Here's how the part is built. I have some questions about the finished solid (model axes, mm). Face numbers are marked on the shaded views. A direction names the side the tool comes from. Give positions to 0.01 mm unless a question says otherwise; leave off trailing zeros. Loops run counter-clockwise (first coordinate to the right, second up) from the corner with the lowest first, then second, coordinate; pieces in that order, holes last. Notation, with made-up numbers: M 78,57 L 123,57 A33 cw 123,89 Z; hole C 35,39.5 d6. An arc over 180 degrees is marked long. Answer as CSV lines item,"result". Start each with the question number.
Item 1: I want a section at A-A on z = 22. List the corners of the cut face in (x, y) for me.
Item 2: If I drill on line 1 along Y through (x, z) = (-90, -13); line 2 along Y through (x, z) = (-90, -21); line 3 along Z through (x, y) = (-107, 9), over which ranges is the centre line in solid material (lowest first)? Write a range as from..to.
Item 3: Will these pins go through, and if not, where does the flat tip stop? P1, Ø1, axis at x = 39.5, z = -3, coming from the +Y side; P2, Ø2, axis at x = 87.5, z = -5, coming from the +Y side; P3, Ø5.5, axis at x = -3.5, z = -17, coming from the +Y side; P4, Ø20, axis at x = 90, y = 50, coming from the +Z side (3 decimals).
Item 4: I want a section at C-C on z = 8. List the corners of the cut face in (x, y) for me, plus the area to 3 significant figures.
Item 5: If we mould it in two halves opening along Y, with no side actions, what happens to the marked faces 3, 4, 5 and 6? For each: released by +Y, released by -Y, zero draft, split by the parting line, or undercut.
Item 6: For the marked faces 1 and 2, which set-ups out of +Z, -Z, +X, -X, +Y, -Y let a thin tool reach every point of the face, with its end or its side?
Item 7: I want a section at B-B on y = 50. List the corners of the cut face in (x, z) for me.
Item 8: I want a section at D-D on y = 68. List the corners of the cut face in (x, z) for me, plus the area to 3 significant figures.
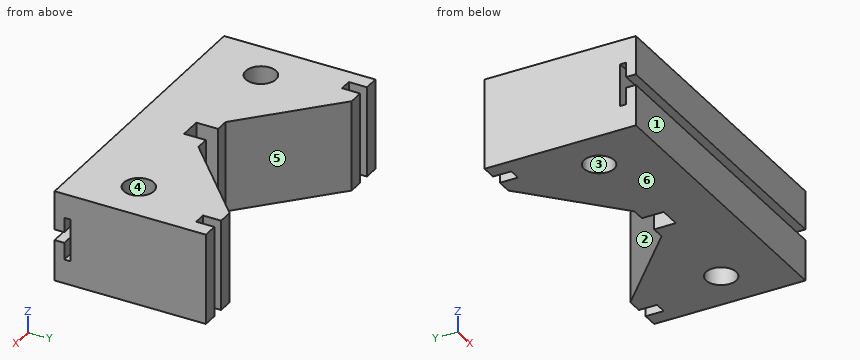
from build123d import *

# Parameters (mm, degrees)
SKETCH2_R           = 12.5
BOSS_EXTRUDE1_DEPTH = 37.5
CUT_EXTRUDE1_DEPTH  = 300


with BuildPart() as part:
    # Sketch2 → Boss-Extrude1 (new body, symmetric)
    with BuildSketch(Plane.XY):
        Polygon((-125, 0), (125, 0), (125, 125), (112.5, 125), (112.5, 110), (102.5, 110), (102.5, 125), (90, 125), (20, 60), (9, 60), (9, 42), (-9, 42), (-9, 60), (-20, 60), (-90, 125), (-102.5, 125), (-102.5, 110), (-112.5, 110), (-112.5, 125), (-125, 125), align=None)
        with Locations((-90, 50)):
            Circle(SKETCH2_R, mode=Mode.SUBTRACT)
        with Locations((90, 50)):
            Circle(SKETCH2_R, mode=Mode.SUBTRACT)
    extrude(amount=BOSS_EXTRUDE1_DEPTH, both=True)

    # Sketch3 → Cut-Extrude1 (cut)
    with BuildSketch(Plane(origin=(125, 0, 0), x_dir=(0, 0, -1), z_dir=(1, 0, 0))):
        Polygon((-17.5, 13), (17.5, 13), (17.5, 8), (3.530117055, 8), (3.530117055, 0), (-5.373528479, 0), (-5.373528479, 8), (-17.5, 8), align=None)
    extrude(amount=-CUT_EXTRUDE1_DEPTH, mode=Mode.SUBTRACT)


solid = part.part
Result:
1,outline,"M -125,0 L 125,0 L 125,125 L 112.5,125 L 112.5,110 L 102.5,110 L 102.5,125 L 90,125 L 20,60 L 9,60 L 9,42 L -9,42 L -9,60 L -20,60 L -90,125 L -102.5,125 L -102.5,110 L -112.5,110 L -112.5,125 L -125,125 Z; hole C -90,50 d25; hole C 90,50 d25"
2,line 1,"0..8, 13..37.5, 62.5..125"
2,line 2,"0..37.5, 62.5..125"
2,line 3,"-37.5..-17.5, 17.5..37.5"
3,P1,"y = 78.57"
3,P2,"y = 123.61"
3,P3,"y = 42"
3,P4,"through"
4,outline,"M -125,0 L 125,0 L 125,8 L -125,8 Z; M -125,13 L 125,13 L 125,125 L 112.5,125 L 112.5,110 L 102.5,110 L 102.5,125 L 90,125 L 20,60 L 9,60 L 9,42 L -9,42 L -9,60 L -20,60 L -90,125 L -102.5,125 L -102.5,110 L -112.5,110 L -112.5,125 L -125,125 Z; hole C -90,50 d25; hole C 90,50 d25"
4,area,"21,200 mm^2"
5,face 3,"undercut"
5,face 4,"undercut"
5,face 5,"released by +Y"
5,face 6,"zero draft"
6,face 1,"+Z, -Z, +X, -X, -Y"
6,face 2,"+Z, -Z, +Y"
7,outline,"M -125,-37.5 L -102.5,-37.5 L -102.5,37.5 L -125,37.5 Z; M -77.5,-37.5 L -9,-37.5 L -9,37.5 L -77.5,37.5 Z; M 9,-37.5 L 77.5,-37.5 L 77.5,37.5 L 9,37.5 Z; M 102.5,-37.5 L 125,-37.5 L 125,37.5 L 102.5,37.5 Z"
8,outline,"M -125,-37.5 L -28.62,-37.5 L -28.62,37.5 L -125,37.5 Z; M 28.62,-37.5 L 125,-37.5 L 125,37.5 L 28.62,37.5 Z"
8,area,"14,500 mm^2"
